Can you work these out from the drawing? Everything is in mm from the part's minimum corner. Round coordinates to 2 decimals unless told otherwise and drop trailing zeros. Order: outer loops, then holes, each group sorted by start corner. A loop starts at its lowest first (then second) coordinate and runs counter-clockwise, first axis right, second up. Notation, with made-up numbers: M 78,70 L 111,70 A5 ccw 111,76 Z; hole C 72,48 d7. An arc over 180 degrees is marked long. Answer as a JSON object with one key per item and string values. Group by question number.
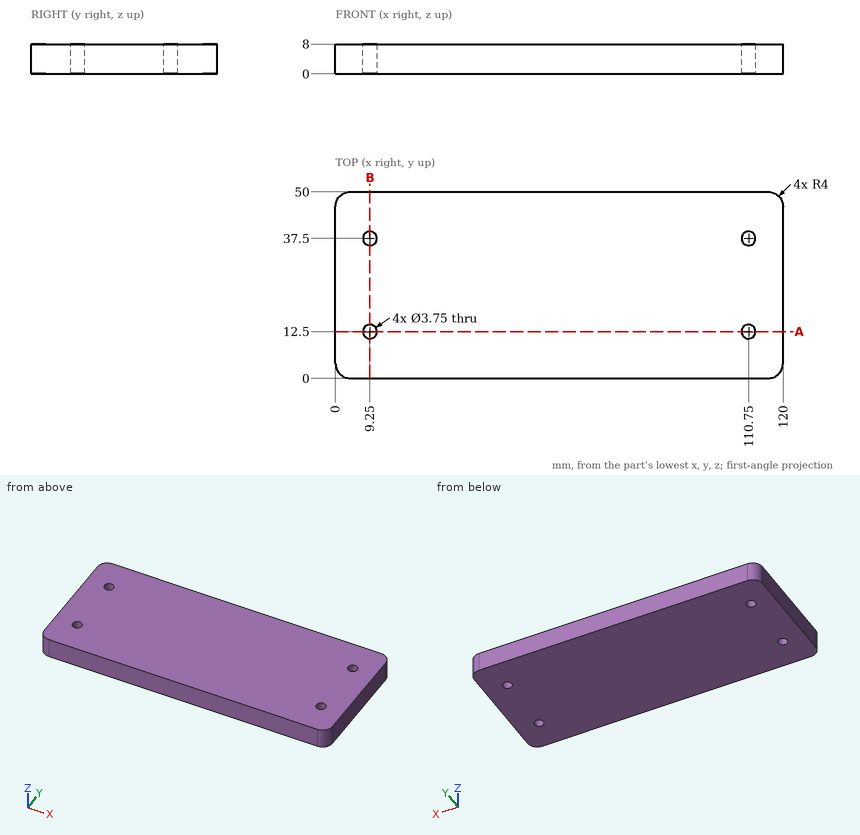
Item 1: Suppose I cut it at A-A, the plane y = 12.5. Write out the boundary of the cut face in (x, z) (3 decimals), and give its area (3 significant figures).
Item 2: I need wall thicknesses on line 1 (Y direction, x = 110.75, z = 4.5) (3 decimals); line 2 (X direction, y = 11, z = 7.25) (3 decimals); line 3 (X direction, y = 37, z = 1.75). Which ranges of each line are inside material? Lowest first, please.
Item 3: Suppose I cut it at B-B, the plane x = 9.25. Write out the boundary of the cut face in (y, z) (3 decimals).
Item 4: I'm going to push a flat-ended pin straight in: pin 1 Ø3 at (x, y) = (110.75, 37.5) entering from +Z. Where does the tip first touch, or does it pass through?
Computed:
{
 "1": {"outline": "M 0,0 L 7.375,0 L 7.375,8 L 0,8 Z; M 11.125,0 L 108.875,0 L 108.875,8 L 11.125,8 Z; M 112.625,0 L 120,0 L 120,8 L 112.625,8 Z", "area": "900 mm^2"},
 "2": {"line 1": "y = 0 to 10.625, 14.375 to 35.625, 39.375 to 50", "line 2": "x = 0 to 8.125, 10.375 to 109.625, 111.875 to 120", "line 3": "x = 0 to 7.44, 11.06 to 108.94, 112.56 to 120"},
 "3": {"outline": "M 0,0 L 10.625,0 L 10.625,8 L 0,8 Z; M 14.375,0 L 35.625,0 L 35.625,8 L 14.375,8 Z; M 39.375,0 L 50,0 L 50,8 L 39.375,8 Z"},
 "4": {"pin 1": "passes through"}
}
